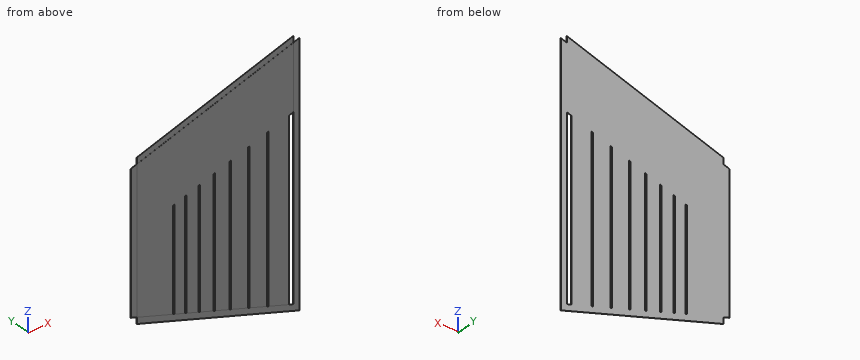
```python
from build123d import *

# Parameters (mm, degrees)
F1_DEPTH = 0.254
F2_DEPTH = 0.127


with BuildPart() as f1:
    # F0 (on Front) → F1 (new body)
    with BuildSketch(Plane.XZ):
        Polygon((-165.1, 96.6560714286), (-165.1, -70.8848640166), (-88.9, -97.3012268737), (-88.9, 120.3325), align=None)
        Polygon((-85.725, 121.3190178571), (-85.725, -98.4019086594), (-63.5, -106.1066811594), (-63.5, 128.2246428571), align=None)
        Polygon((-60.325, 129.2111607143), (-60.325, -107.2073629451), (-34.925, -116.0128172308), (-34.925, 137.1033035714), align=None)
        Polygon((-31.75, 138.0898214286), (-31.75, -117.1134990166), (-3.175, -127.019635088), (-3.175, 146.9684821429), align=None)
        Polygon((0, 147.955), (0, -128.1203168737), (30.1625, -138.576793838), (30.1625, 157.3269196429), align=None)
        Polygon((33.3375, -139.6774756237), (69.85, -152.3353161594), (69.85, 169.6583928571), (33.3375, 158.3134375), align=None)
        Polygon((112.7125, -167.1945202666), (155.575, -182.0537243737), (155.575, 196.294375), (112.7125, 182.9763839286), align=None)
        Polygon((73.025, -153.4359979451), (109.5375, -166.0938384808), (109.5375, 181.9898660714), (73.025, 170.6449107143), align=None)
        Polygon((-165.1, 235.7571436628), (-165.1, 96.6560714286), (-88.9, 120.3325), (-85.725, 121.3190178571), (-63.5, 128.2246428571), (-60.325, 129.2111607143), (-34.925, 137.1033035714), (-31.75, 138.0898214286), (-3.175, 146.9684821429), (0, 147.955), (30.1625, 157.3269196429), (33.3375, 158.3134375), (69.85, 169.6583928571), (73.025, 170.6449107143), (109.5375, 181.9898660714), (112.7125, 182.9763839286), (155.575, 196.294375), (158.75, 197.2808928571), (165.1, 199.2539285714), (165.1, 338.3550008057), align=None)
    extrude(amount=F1_DEPTH)

    # F0 (on Front) → F2 (join)
    with BuildSketch(Plane.XZ):
        Polygon((-177.8, 231.8110722342), (-177.8, 92.71), (-165.1, 96.6560714286), (-165.1, 235.7571436628), align=None)
        Polygon((-165.1, 249.0560714286), (-165.1, 235.7571436628), (165.1, 338.3550008057), (165.1, 351.6539285714), align=None)
        Polygon((177.8, 342.3010722342), (165.1, 338.3550008057), (165.1, 199.2539285714), (177.8, 203.2), align=None)
        Polygon((-177.8, 92.71), (-177.8, 0), (-177.8, -66.4821368737), (-165.1, -70.8848640166), (-165.1, 96.6560714286), align=None)
        Polygon((-88.9, -97.3012268737), (-165.1, -70.8848640166), (-165.1, -84.3263671429), (155.575, -195.4952275), (155.575, -182.0537243737), (112.7125, -167.1945202666), (109.5375, -166.0938384808), (73.025, -153.4359979451), (69.85, -152.3353161594), (33.3375, -139.6774756237), (30.1625, -138.576793838), (0, -128.1203168737), (-3.175, -127.019635088), (-31.75, -117.1134990166), (-34.925, -116.0128172308), (-60.325, -107.2073629451), (-63.5, -106.1066811594), (-85.725, -98.4019086594), align=None)
        Polygon((177.8, 203.2), (165.1, 199.2539285714), (165.1, -185.3557697308), (177.8, -189.7584968737), (177.8, 0), align=None)
        Polygon((155.575, -182.0537243737), (155.575, -195.4952275), (165.1, -198.7972728571), (165.1, -185.3557697308), (158.75, -183.1544061594), align=None)
        Polygon((165.1, -185.3557697308), (165.1, -198.7972728571), (177.8, -203.2), (177.8, -189.7584968737), align=None)
    extrude(amount=F2_DEPTH)


solid = f1.part
```
For this review, take the finished solid that the model builds, in its own axes (mm). Round coordinates to 2 decimals unless told otherwise and drop trailing zeros. Write each loop counter-clockwise with the first axis right and the second up, starting at its lowest first coordinate (ties: lowest second). Pieces come first, ordered by that corner, then holes. Notation, with made-up numbers: (11.5, 43) - (50.5, 43) arc R8 cw to (50.5, 58) - close; hole circle Ø11 at (-21.5, 15). An arc over 180 degrees is marked (long way). Answer as CSV lines item,"result". Start each with the question number.
(1) Add section B-B, the plane x = 134. State the section outline as (y, z) points.
(2) For line 1 (X direction, y = -0.05, z = 238.5); line 2 (Z direction, x = 33, y = -0.05); line 3 (Z direction, x = -60, y = -0.2), list the stretches that pass through material, from the lowest coordinate up.
(3) Add section A-A, the plane z = 71. State how many separate pieces and enclosed holes the cut face has, plus the area to 3 significant figures.
(4) Add section C-C, the plane x = -43. State the section outline as (y, z) points.
(5) For pin 1 (1 mm diameter, centred on x = -65, z = -118.5, fed in from -Y), flat-tipped, find the tip position at first contact; note if it passes through.
From the geometry:
1,outline,"(-0.25, -174.57) - (-0.13, -174.57) - (-0.13, -188.02) - (0, -188.02) - (0, 341.99) - (-0.13, 341.99) - (-0.13, 328.69) - (-0.25, 328.69) - close"
2,line 1,"x = -165.1 to 177.8"
2,line 2,"z = -153 to -139.56, 158.21 to 310.61"
2,line 3,"z = -107.32 to 268.41"
3,separate pieces,"9"
3,enclosed holes,"0"
3,area,"79.0 mm²"
4,outline,"(-0.25, -113.21) - (-0.13, -113.21) - (-0.13, -126.65) - (0, -126.65) - (0, 286.99) - (-0.13, 286.99) - (-0.13, 273.7) - (-0.25, 273.7) - close"
5,pin 1,"stops at y = -0.13"
